Could you check a few things on this drawing? It's one solid part, dimensions in mm from its lowest x, y, z. A direction names the side the tool comes from. Round coordinates to 2 decimals unless told otherwise and drop trailing zeros. Write each loop counter-clockwise with the first axis right and the second up, starting at its lowest first coordinate (ties: lowest second). Pieces come first, ordered by that corner, then holes. Notation, with made-up numbers: (48.5, 0.25) -> (90.5, 0.25) arc R37 cw to (90.5, 38.25) -> close; hole circle Ø6 at (62.5, 37). An arc over 180 degrees is marked (long way). Answer as CSV lines item,"result".
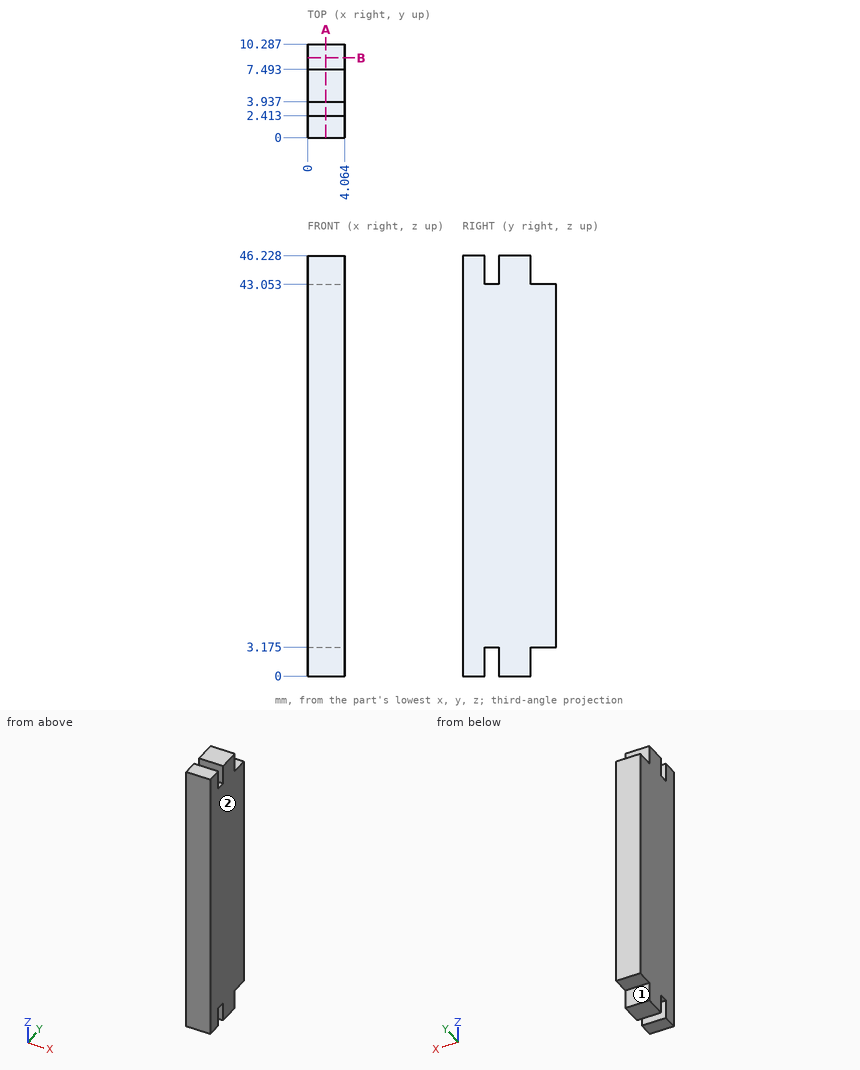
1. Suppose I cut it at A-A on x = 2. Please give me the cut outline in (y, z) (3 decimals), and give its area (3 significant figures).
Numbers:
outline,"(0, 0) -> (2.413, 0) -> (2.413, 3.175) -> (3.937, 3.175) -> (3.937, 0) -> (7.493, 0) -> (7.493, 3.175) -> (10.287, 3.175) -> (10.287, 43.053) -> (7.493, 43.053) -> (7.493, 46.228) -> (3.937, 46.228) -> (3.937, 43.053) -> (2.413, 43.053) -> (2.413, 46.228) -> (0, 46.228) -> close"
area,"448 mm^2"
2. Suppose I cut it at B-B on y = 8.75. Please give me the cut outline in (x, z) (3 decimals), and give its area (3 significant figures).
Numbers:
outline,"(0, 3.175) -> (4.064, 3.175) -> (4.064, 43.053) -> (0, 43.053) -> close"
area,"162 mm^2"
3. On a 3-axis mill with a long thin cutter (end or side, diameter ignored), from which of +Z, -Z, +X, -X, +Y, -Y can I reach the whole of each face in a straight line? I mean the marked faces 1 and 2. Say none if no direction works.
Numbers:
face 1,"-Z, +X, -X, +Y"
face 2,"+Z, -Z, +X, +Y, -Y"
4. For pin 1 Ø0.5 at (x, y) = (2, 3) entering from -Z (3 decimals); pin 2 Ø1 at (x, z) = (2, 45.5) entering from +Y; pin 3 Ø1 at (x, z) = (1, 44) entering from -Y; pin 4 Ø0.8 at (x, y) = (2, 9) entering from +Z, each with a flat end and sliding along its axis, tell me the tip position at first contact or that it passes through.
Numbers:
pin 1,"stops at z = 3.175"
pin 2,"stops at y = 7.49"
pin 3,"stops at y = 0"
pin 4,"stops at z = 43.05"
5. If I drill on line 1 (Z direction, x = 2.95, y = 8) (3 decimals), over which ranges is the centre line in solid material (lowest first)?
Numbers:
line 1,"z = 3.175 to 43.053"
